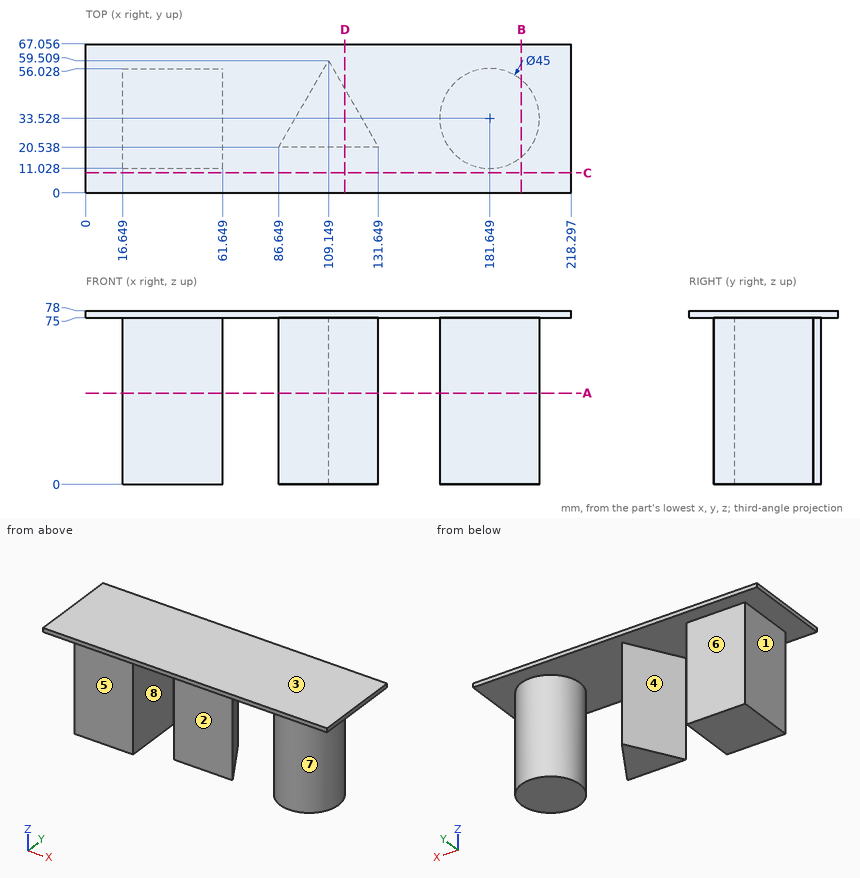
Input: dimensioned drawing with shaded views. Units: mm. Origin: part minimum x, y, z. A direction names the side the tool comes from. Coordinates: 2 decimals unless noted, no trailing zeros. Order: outer loops, then holes, each group sorted by start corner. A loop starts at its lowest first (then second) coordinate and runs counter-clockwise, first axis right, second up. Notation, with made-up numbers: (82.5, 13) - (109.5, 13) arc R10 ccw to (109.5, 18) - close; hole circle Ø3 at (64, 3). An arc over 180 degrees is marked (long way). Return JSON: item names as keys, results as strings. Group by question number.
1. Cut plane C-C (y = 9). Output: boundary loops of the cut face in (x, z).
2. Set-up query: the marked faces 4, 5, 6, 7 and 8. Return all of +Z, -Z, +X, -X, +Y, -Y with unobstructed straight access to the full face (end or side cutting, diameter ignored); none if empty.
3. Cut plane B-B (x = 196). Output: boundary loops of the cut face in (y, z) (1 decimal).
4. Material intervals for line 1 along Y through (x, z) = (48.5, 8); line 2 along Z through (x, y) = (124.5, 35.5); line 3 along Y through (x, z) = (194, 56) (1 decimal), sorted ascending. Write a range as [from, to].
5. Pull-direction query (X, two-part tool) for the marked faces 1, 2 and 3; classes: pulls with the +X half, pulls with the -X half, needs draft (parallel to the pull), parting line crosses it, or undercut.
6. Cut plane D-D (x = 116.5). Output: boundary loops of the cut face in (y, z) (1 decimal).
7. Cut plane A-A (z = 41). Output: boundary loops of the cut face in (x, y).
8. Pin query (flat end, axial travel): pin 1 (8 mm diameter, centred on x = 177, z = 62, fed in from +Y); pin 2 (13.5 mm diameter, centred on y = 43, z = 52, fed in from -X); pin 3 (1.5 mm diameter, centred on y = 28.5, z = 25, fed in from +X); pin 4 (20 mm diameter, centred on x = 92.5, y = 50, fed in from -Z). Return the tip coordinate at first contact, or that it passes through.
Resolved:
{
 "1": {"outline": "(0, 75) - (218.3, 75) - (218.3, 78) - (0, 78) - close"},
 "2": {"face 4": "-Z, +Y", "face 5": "-Z, +X, -X, -Y", "face 6": "-Z, -X, +Y", "face 7": "-Z", "face 8": "-Z, +Y, -Y"},
 "3": {"outline": "(0, 75) - (16.2, 75) - (16.2, 0) - (50.9, 0) - (50.9, 75) - (67.1, 75) - (67.1, 78) - (0, 78) - close"},
 "4": {"line 1": "y = [11.03, 56.03]", "line 2": "z = [75, 78]", "line 3": "y = [14.7, 52.3]"},
 "5": {"face 1": "pulls with the -X half", "face 2": "undercut", "face 3": "needs draft"},
 "6": {"outline": "(0, 75) - (20.5, 75) - (20.5, 0) - (46.8, 0) - (46.8, 75) - (67.1, 75) - (67.1, 78) - (0, 78) - close"},
 "7": {"outline": "(16.65, 11.03) - (61.65, 11.03) - (61.65, 56.03) - (16.65, 56.03) - close; (86.65, 20.54) - (131.65, 20.54) - (109.15, 59.51) - close; circle Ø45 at (181.65, 33.53)"},
 "8": {"pin 1": "stops at y = 56.02", "pin 2": "stops at x = 16.65", "pin 3": "stops at x = 203.74", "pin 4": "stops at z = 0"}
}
